For this review, take the finished solid that the model builds, in its own axes (mm). A direction names the side the tool comes from. Coordinates: 2 decimals unless noted, no trailing zeros. Loops run counter-clockwise (first coordinate to the right, second up) from the corner with the lowest first, then second, coordinate; pieces in that order, holes last. Notation, with made-up numbers: (17, 63.25) -> (52, 63.25) arc R20 cw to (52, 85.25) -> close; hole circle Ø3 at (-5, 57.5). An arc over 180 degrees is marked (long way). One line per item, written item: value.
from build123d import *

# Parameters (mm, degrees)
F0_R     = 3.175
F1_DEPTH = 6.35
F2_W     = 6.35
F2_H     = 25.4
F3_DEPTH = 81.28
F4_W     = 234.95
F4_H     = 25.4
F4_W_2   = 6.35
F5_DEPTH = 6.35
F6_R     = 3.175
F7_DEPTH = 508


with BuildPart() as f1:
    # F0 (on Front) → F1 (new body)
    with BuildSketch(Plane.XZ):
        Polygon((0, 12.7), (0, 0), (241.3, 0), (241.3, 12.7), (241.3, 25.4), (120.65, 25.4), (0, 25.4), align=None)
        with BuildLine():
            ThreePointArc((22.225, 12.7), (19.05, 9.525), (15.875, 12.7))
            ThreePointArc((15.875, 12.7), (19.05, 15.875), (22.225, 12.7))
        make_face(mode=Mode.SUBTRACT)
        with BuildLine():
            ThreePointArc((123.825, 12.7), (118.404936, 10.454936), (120.65, 15.875))
            ThreePointArc((120.65, 15.875), (122.895064, 14.945064), (123.825, 12.7))
        make_face(mode=Mode.SUBTRACT)
        with Locations((222.25, 12.7)):
            Circle(F0_R, mode=Mode.SUBTRACT)
    extrude(amount=F1_DEPTH)

    # F2 (on face) → F3 (join)
    with BuildSketch(Plane.XZ.offset(6.35)):
        with Locations((3.175, 12.7)):
            Rectangle(F2_W, F2_H)
        with Locations((238.125, 12.7)):
            Rectangle(F2_W, F2_H)
    extrude(amount=F3_DEPTH)

    # F4 (on face) → F5 (join)
    with BuildSketch(Plane.XZ.offset(87.63)):
        with Locations((123.825, 12.7)):
            Rectangle(F4_W, F4_H)
        with Locations((3.175, 12.7)):
            Rectangle(F4_W_2, F4_H)
    extrude(amount=F5_DEPTH)

    # F6 (on face) → F7 (cut)
    with BuildSketch(Plane.XZ.offset(6.35)):
        with Locations((222.25, 12.7)):
            Circle(F6_R)
        with Locations((120.65, 12.7)):
            Circle(F6_R)
        with Locations((19.05, 12.7)):
            Circle(F6_R)
    extrude(amount=F7_DEPTH, mode=Mode.SUBTRACT)


solid = f1.part
1. Take a section at B-B, the plane x = 207. Give the boundary of the cut face in (y, z).
Return value:
outline: (-93.98, 0) -> (-87.63, 0) -> (-87.63, 25.4) -> (-93.98, 25.4) -> close; (-6.35, 0) -> (0, 0) -> (0, 25.4) -> (-6.35, 25.4) -> close
2. To check wall thickness, follow probe 1 along X at (y, z) = (-91, 12.7) (3 decimals); probe 2 along Y at (x, z) = (188, 2); probe 3 along X at (y, z) = (-56, 22.5). State the ranges of each line that lie inside material, in increasing order. Write a range as from..to.
Return value:
probe 1: x = 0..15.875, 22.225..117.475, 123.825..219.075, 225.425..241.3
probe 2: y = -93.98..-87.63, -6.35..0
probe 3: x = 0..6.35, 234.95..241.3
3. Take a section at A-A, the plane y = -50. Give the boundary of the cut face in (x, z).
Return value:
outline: (0, 0) -> (6.35, 0) -> (6.35, 25.4) -> (0, 25.4) -> close; (234.95, 0) -> (241.3, 0) -> (241.3, 25.4) -> (234.95, 25.4) -> close
4. Take a section at C-C, the plane z = 3.75. Give the boundary of the cut face in (x, y).
Return value:
outline: (0, -93.98) -> (241.3, -93.98) -> (241.3, 0) -> (0, 0) -> close; hole (6.35, -87.63) -> (234.95, -87.63) -> (234.95, -6.35) -> (6.35, -6.35) -> close
5. For faces 1 (the cylindrical face through (16.02, -3.13, 13.65)), 2 (the flat face through (119, -87.63, 16)), list the 3-axis set-ups (+Z, -Z, +X, -X, +Y, -Y) from which the entire face can be reached by the end or side of a thin tool; tool diameter is ignored.
Return value:
face 1: +Y, -Y
face 2: +Z, -Z
6. The part is to be moulded in two halves that separate along X. For faces 3 (the flat face through (6.35, -46, 13)), 4 (the flat face through (119, 0, 16)), 5 (the flat face through (0, -46, 13)), say which applies: pulls with the +X half, pulls with the -X half, needs draft (parallel to the pull), parting line crosses it, or undercut.
Return value:
face 3: undercut
face 4: needs draft
face 5: pulls with the -X half
